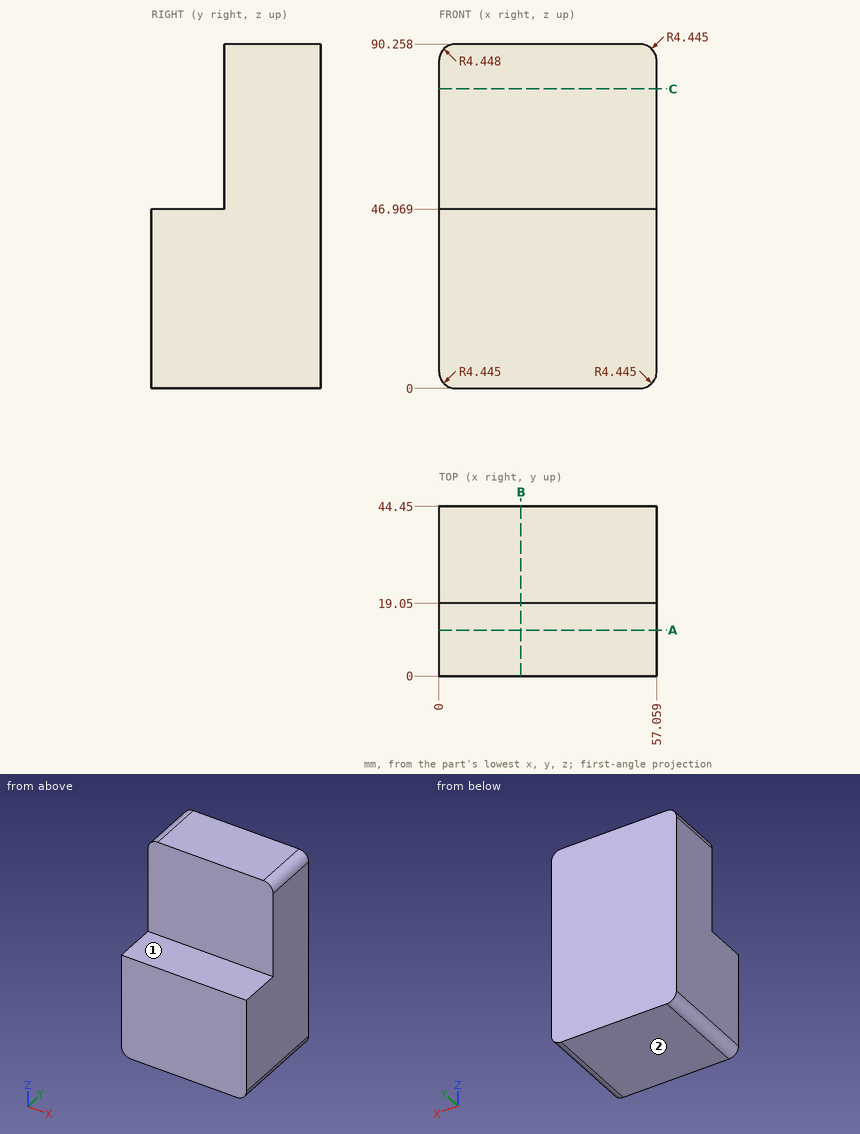
Design review of the part shown in the three views and the two pictorial views. Dimensions are in mm from the part's minimum x, y and z. A direction names the side the tool comes from. Give positions to 0.01 mm unless a question says otherwise; leave off trailing zeros. Write each loop counter-clockwise with the first axis right and the second up, starting at its lowest first coordinate (ties: lowest second). Pieces come first, ordered by that corner, then holes. Notation, with made-up numbers: M -35.75,-25.5 L 1.25,-25.5 A12 cw 1.25,-16.5 Z; hole C 83,-22 d7. An arc over 180 degrees is marked long. Answer in a Markdown table with one row per item.
Item 1: Add section A-A on y = 12. Give the boundary of the cut face in (x, z) (1 decimal).
Check sheet entries:
| item | result |
|---|---|
| outline | M 0,4.4 A4.4 ccw 4.4,0 L 52.6,0 A4.4 ccw 57.1,4.4 L 57.1,47 L 0,47 Z |
Item 2: Tool access review of the marked faces 1 and 2: name each direction out of +Z, -Z, +X, -X, +Y, -Y from which nothing blocks a thin tool from reaching the whole face with its end or side.
Check sheet entries:
| item | result |
|---|---|
| face 1 | +Z, +X, -X, -Y |
| face 2 | -Z, +X, -X, +Y, -Y |
Item 3: For line 1 along Y through (x, z) = (4, 78); line 2 along Z through (x, y) = (8.5, 11); line 3 along Z through (x, y) = (3, 31) (1 decimal), list the stretches that pass through material, from the lowest coordinate up.
Check sheet entries:
| item | result |
|---|---|
| line 1 | 19.05 to 44.45 |
| line 2 | 0 to 46.97 |
| line 3 | 0.2 to 90 |
Item 4: For P1, Ø1.5, axis at x = 50.5, y = 17.5, coming from the +Z side; P2, Ø12, axis at x = 21.5, z = 75, coming from the -Y side, all flat-tipped, find the tip position at first contact; note any pin that passes through.
Check sheet entries:
| item | result |
|---|---|
| P1 | z = 46.97 |
| P2 | y = 19.05 |
Item 5: Add section B-B on x = 21.5. Give the boundary of the cut face in (y, z).
Check sheet entries:
| item | result |
|---|---|
| outline | M 0,0 L 44.45,0 L 44.45,90.26 L 19.05,90.26 L 19.05,46.97 L 0,46.97 Z |
Item 6: Add section C-C on z = 78.5. Give the boundary of the cut face in (x, y), plus the area to 3 significant figures.
Check sheet entries:
| item | result |
|---|---|
| outline | M 0,19.05 L 57.06,19.05 L 57.06,44.45 L 0,44.45 Z |
| area | 1,450 mm2 |
